Work out the finished part from the listing and answer in its coordinate system (mm). Give positions to 0.01 mm unless a question says otherwise; leave off trailing zeros. Loops run counter-clockwise (first coordinate to the right, second up) from the corner with the lowest first, then second, coordinate; pieces in that order, holes last. Notation, with made-up numbers: M 0.25,65 L 41.25,65 A23 ccw 41.25,93 Z; hole C 86,57 d11. An arc over 180 degrees is marked long. Use a Markdown table: item, result.
```python
from build123d import *

# Parameters (mm, degrees)
SKETCH1_W                    = 1206.5
SKETCH1_H                    = 596.9
BOSS_EXTRUDE1_DEPTH          = 17.78
FILLET1_R                    = 6.35
SKETCH4_W                    = 165.1
SKETCH4_H                    = 69.85
SKETCH4_W_2                  = 114.3
SKETCH4_H_2                  = 152.4
CUT_EXTRUDE1_DEPTH           = 18.78
FILLET2_R                    = 6.35
F_1_8_0_125_DIAMETER_HOLE2_D = 3.175


with BuildPart() as part:
    # Sketch1 → Boss-Extrude1 (new body)
    with BuildSketch(Plane(origin=(0, 0, 0), x_dir=(1, 0, 0), z_dir=(0, 1, 0))):
        Rectangle(SKETCH1_W, SKETCH1_H)
    extrude(amount=BOSS_EXTRUDE1_DEPTH)

    # Fillet1
    fillet1_edges = [part.edges().sort_by_distance(p)[0] for p in [
        (603.25, 8.89, 298.45),
        (-603.25, 8.89, 298.45),
        (-603.25, 8.89, -298.45),
        (603.25, 8.89, -298.45),
    ]]
    fillet(fillet1_edges, radius=FILLET1_R)

    # Sketch4 → Cut-Extrude1 (cut, through all)
    with BuildSketch(Plane(origin=(0, 17.78, 0), x_dir=(1, 0, 0), z_dir=(0, 1, 0))):
        with Locations((0, -263.525)):
            Rectangle(SKETCH4_W, SKETCH4_H)
        with Locations((-546.1, 0)):
            Rectangle(SKETCH4_W_2, SKETCH4_H_2)
        with Locations((546.1, 0)):
            Rectangle(SKETCH4_W_2, SKETCH4_H_2)
    extrude(amount=-CUT_EXTRUDE1_DEPTH, mode=Mode.SUBTRACT)

    # Fillet2
    fillet2_edges = [part.edges().sort_by_distance(p)[0] for p in [
        (82.55, 8.89, 228.6),
        (82.55, 8.89, 298.45),
        (-82.55, 8.89, 298.45),
        (-82.55, 8.89, 228.6),
        (-603.25, 8.89, 76.2),
        (-603.25, 8.89, -76.2),
        (-488.95, 8.89, -76.2),
        (-488.95, 8.89, 76.2),
        (603.25, 8.89, -76.2),
        (603.25, 8.89, 76.2),
        (488.95, 8.89, 76.2),
        (488.95, 8.89, -76.2),
    ]]
    fillet(fillet2_edges, radius=FILLET2_R)

    # 1/8 (0.125) Diameter Hole2 (through all)
    with Locations(Plane(origin=(0, 0, 0), x_dir=(-1, 0, 0), z_dir=(0, -1, 0))):
        with Locations((-439.865615282, 175.258956089), (439.865615282, 175.258956089), (439.865615282, -175.258956089), (0, 0), (-439.865615282, -175.258956089)):
            Hole(F_1_8_0_125_DIAMETER_HOLE2_D / 2)


solid = part.part
```
(1) A cutting plane is placed at B-B (y = 6.75). Count the separate pieces of the cut face and the enclosed holes in it, and give its area (3 significant figures).
Entries:
| item | result |
|---|---|
| separate pieces | 1 |
| enclosed holes | 5 |
| area | 674,000 mm² |
(2) Consider probe 1 along Z at (x, y) = (0, 11.5); probe 2 along Z at (x, y) = (554.5, 10.75); probe 3 along X at (y, z) = (3.5, -50). Determine where each line is inside the solid, lowest interval first. Write a range as [from, to].
Entries:
| item | result |
|---|---|
| probe 1 | z = [-298.45, -1.59], [1.59, 228.6] |
| probe 2 | z = [-298.45, -76.2], [76.2, 298.45] |
| probe 3 | x = [-488.95, 488.95] |
(3) A cutting plane is placed at A-A (z = -46). Write down the section's boundary in (x, y), and give its area (3 significant figures).
Entries:
| item | result |
|---|---|
| outline | M -488.95,0 L 488.95,0 L 488.95,17.78 L -488.95,17.78 Z |
| area | 17,400 mm² |
(4) Given P1, Ø5.5, axis at y = 11.5, z = -29.5, coming from the +X side; P2, Ø3, axis at x = -439.87, z = -175.26, coming from the +Y side, each flat-ended and moving along its own axis, determine where each tip first touches the part or whether it passes through.
Entries:
| item | result |
|---|---|
| P1 | stops at x = 488.95 |
| P2 | passes through |
